Could you check a few things on this drawing? It's one solid part, dimensions in mm from its lowest x, y, z. A direction names the side the tool comes from. Give positions to 0.01 mm unless a question says otherwise; leave off trailing zeros. Loops run counter-clockwise (first coordinate to the right, second up) from the corner with the lowest first, then second, coordinate; pieces in that order, holes last.
Q1. Suppose I cut it at C-C (y = 3.5). List the corners of the cut face in (x, z) for me, and give its area (3 significant figures).
Q2. I'm going to push flat-ended pins straight in: P1, Ø1.5, axis at y = 6, z = 39.5, coming from the +X side; P2, Ø4, axis at x = 95.5, y = 5.5, coming from the +Z side; P3, Ø1.5, axis at x = 79.5, y = 6, coming from the +Z side. Where does each tip first touch, or does it pass through?
Q3. Thinking about a two-plate mould opening in X: for the marked faces 1 and 2, which applies, pulls with the +X half, pulls with the -X half, needs draft (parallel to the pull), parting line crosses it, or undercut?
Q4. Suppose I cut it at D-D (z = 30). List the corners of the cut face in (x, y) for me, and give its area (3 significant figures).
Q5. Suppose I cut it at B-B (x = 80). List the corners of the cut face in (y, z) for me.
Q6. Suppose I cut it at A-A (z = 55). List the corners of the cut face in (x, y) for me, and give its area (3 significant figures).
Q7. I need wall thicknesses on probe 1 along Z at (x, y) = (55, 2.5); probe 2 along X at (y, z) = (5.5, 76); probe 3 along X at (y, z) = (6.75, 81). Which ranges of each line are inside material? Lowest first, please.
Q8. For the marked faces 3 and 4, which set-ups out of +Z, -Z, +X, -X, +Y, -Y let a thin tool reach every point of the face, with its end or its side?
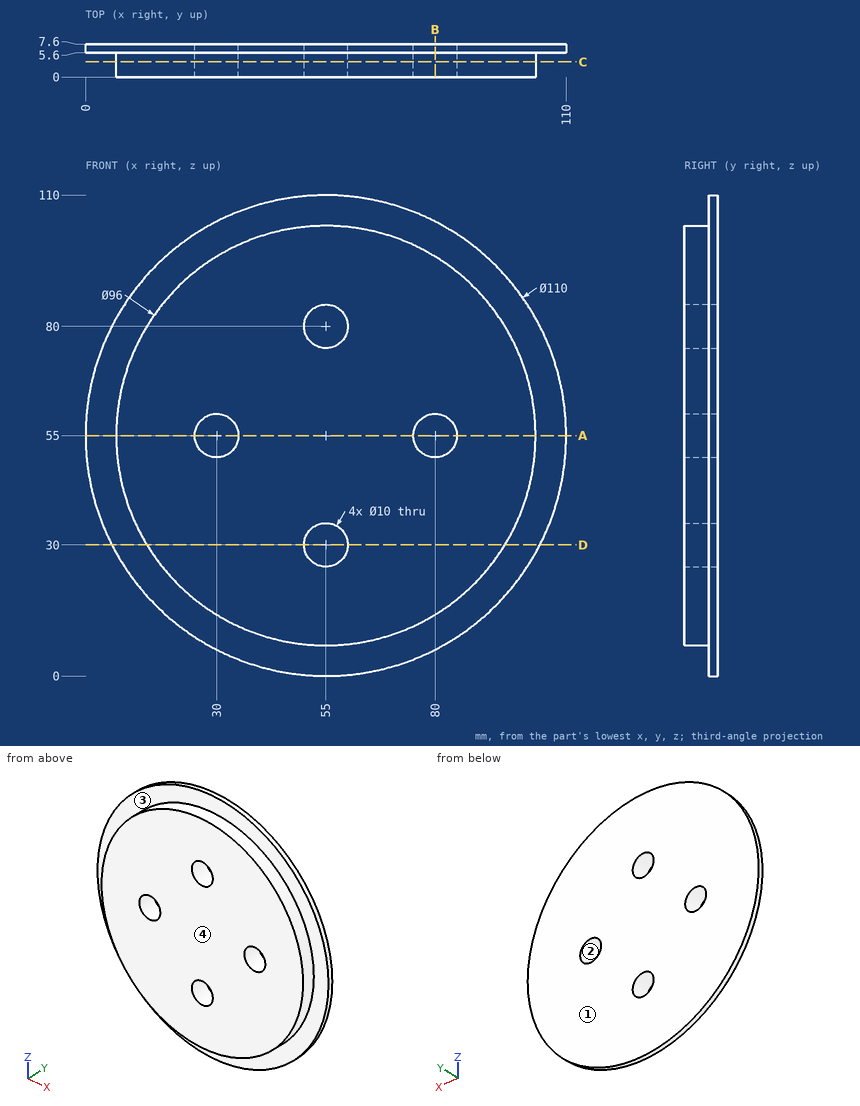
Solutions:
1. outline: circle Ø96 at (55, 55); hole circle Ø10 at (30, 55); hole circle Ø10 at (55, 30); hole circle Ø10 at (55, 80); hole circle Ø10 at (80, 55)
1. area: 6,920 mm2
2. P1: stops at x = 107.99
2. P2: stops at z = 94.28
2. P3: stops at z = 104.61
3. face 1: needs draft
3. face 2: undercut
4. outline: (6.01, 5.6) - (14.02, 5.6) - (14.02, 0) - (50, 0) - (50, 7.6) - (6.01, 7.6) - close; (60, 0) - (95.98, 0) - (95.98, 5.6) - (103.99, 5.6) - (103.99, 7.6) - (60, 7.6) - close
4. area: 579 mm2
5. outline: (0, 14.02) - (5.6, 14.02) - (5.6, 6.01) - (7.6, 6.01) - (7.6, 50) - (0, 50) - close; (0, 60) - (7.6, 60) - (7.6, 103.99) - (5.6, 103.99) - (5.6, 95.98) - (0, 95.98) - close
6. outline: (0, 5.6) - (7, 5.6) - (7, 0) - (25, 0) - (25, 7.6) - (0, 7.6) - close; (35, 0) - (75, 0) - (75, 7.6) - (35, 7.6) - close; (85, 0) - (103, 0) - (103, 5.6) - (110, 5.6) - (110, 7.6) - (85, 7.6) - close
6. area: 606 mm2
7. probe 1: z = 7 to 25, 35 to 75, 85 to 103
7. probe 2: x = 11.84 to 52, 58 to 98.16
7. probe 3: x = 6.53 to 50.1, 59.9 to 103.47
8. face 3: -Y
8. face 4: +Z, -Z, +X, -X, -Y
